from build123d import *

# Parameters (mm, degrees)
SKETCH1_W                      = 81.37
SKETCH1_H                      = 20
SKETCH1_R                      = 2.5
BOSS_EXTRUDE1_DEPTH            = 15
CBORE_FOR_M5_SHCS1_D           = 5.5
CBORE_FOR_M5_SHCS1_CBORE_D     = 10
CBORE_FOR_M5_SHCS1_CBORE_DEPTH = 10
SKETCH8_W                      = 20
SKETCH8_H                      = 15
BOSS_EXTRUDE3_DEPTH            = 8.5
CUT_EXTRUDE1_START             = -3
CUT_EXTRUDE1_DEPTH             = 9
SKETCH7_W                      = 5
SKETCH7_H                      = 6.1
BOSS_EXTRUDE2_DEPTH            = 4
CHAMFER1_SIZE                  = 0.5


with BuildPart() as part:
    # Sketch1 → Boss-Extrude1 (new body)
    with BuildSketch(Plane(origin=(0, 0, 0), x_dir=(1, 0, 0), z_dir=(0, 1, 0))):
        with Locations((-29.315, 0)):
            Rectangle(SKETCH1_W, SKETCH1_H)
        Circle(SKETCH1_R, mode=Mode.SUBTRACT)
        with Locations((-18.03, 0)):
            Circle(SKETCH1_R, mode=Mode.SUBTRACT)
    extrude(amount=BOSS_EXTRUDE1_DEPTH)

    # CBORE for M5 SHCS1 (through all)
    with Locations(Plane(origin=(0, 15, 0), x_dir=(1, 0, 0), z_dir=(0, 1, 0))):
        with Locations((-58, 0), (-38.03, 0)):
            CounterBoreHole(CBORE_FOR_M5_SHCS1_D / 2, CBORE_FOR_M5_SHCS1_CBORE_D / 2, CBORE_FOR_M5_SHCS1_CBORE_DEPTH)

    # Sketch8 → Boss-Extrude3 (add)
    with BuildSketch(Plane(origin=(11.37, 0, 0), x_dir=(0, 0, -1), z_dir=(1, 0, 0))):
        with Locations((0, 7.5)):
            Rectangle(SKETCH8_W, SKETCH8_H)
    extrude(amount=BOSS_EXTRUDE3_DEPTH)

    # Sketch6 → Cut-Extrude1 (cut)
    with BuildSketch(Plane(origin=(0, 15, 0), x_dir=(1, 0, 0), z_dir=(0, 1, 0)).offset(CUT_EXTRUDE1_START)):
        with BuildLine():
            Line((-29.53, 0), (-29.53, -10))
            Line((-29.53, -10), (11.5, -10))
            Line((11.5, -10), (11.5, 0))
            ThreePointArc((11.5, 0), (3.780046296, 10.860996731), (-9.015, 7.140012255))
            ThreePointArc((-9.015, 7.140012255), (-21.810046296, 10.860996731), (-29.53, 0))
        make_face()
    extrude(amount=-CUT_EXTRUDE1_DEPTH, mode=Mode.SUBTRACT)

    # Sketch7 → Boss-Extrude2 (add)
    with BuildSketch(Plane.XZ):
        with Locations((-11.5, 0)):
            Rectangle(SKETCH7_W, SKETCH7_H)
        with Locations((-67.5, 0)):
            Rectangle(SKETCH7_W, SKETCH7_H)
    extrude(amount=BOSS_EXTRUDE2_DEPTH)

    # Chamfer1
    chamfer1_edges = [part.edges().sort_by_distance(p)[0] for p in [
        (-2.5, 15, 0),
        (-70, 15, 0),
        (-20.53, 15, 0),
        (-25.065, 15, 10),
        (-43.03, 15, 0),
        (-63, 15, 0),
        (19.87, 15, 0),
        (-25.065, 15, -10),
    ]]
    chamfer(chamfer1_edges, length=CHAMFER1_SIZE)


solid = part.part
The model under review builds one solid part; all positions refer to its coordinate system, in mm. A direction names the side the tool comes from. Round coordinates to 2 decimals unless told otherwise and drop trailing zeros. Loops run counter-clockwise (first coordinate to the right, second up) from the corner with the lowest first, then second, coordinate; pieces in that order, holes last. Notation, with made-up numbers: M 80,29.25 L 108,29.25 A15 ccw 108,48.25 Z; hole C -15.5,20 d2. An arc over 180 degrees is marked long. Answer as a JSON object with one key per item and string values.
Item 1: Clearance check with flat-ended pins moving along their axes: P1, Ø2, axis at x = -37.5, z = -7.5, coming from the -Y side; P2, Ø4.5, axis at x = -58, z = 0, coming from the +Y side; P3, Ø5, axis at x = -38.5, z = -1.5, coming from the +Y side; P4, Ø3, axis at x = -12.5, y = -2.5, coming from the +Z side. State where each tip first meets the part, or that it passes through.
Check sheet entries:
{"P1": "y = 0", "P2": "through", "P3": "y = 5", "P4": "z = 3.05"}
Item 2: For line 1 along X through (y, z) = (13.55, 0); line 2 along X through (y, z) = (-1.25, -1.5); line 3 along Z through (x, y) = (-18.03, 2.25), list the stretches that pass through material, from the lowest coordinate up.
Check sheet entries:
{"line 1": "-70 to -63, -53 to -43.03, -33.03 to -20.53, -15.53 to -2.5, 2.5 to 19.87", "line 2": "-70 to -65, -14 to -9", "line 3": "-10 to -2.5, 2.5 to 10"}
Item 3: The part is to be moulded in two halves that separate along Y. For faces 1 (the face through (11.5, 8, 5)), 2 (the face through (-10.52, 7.56, -8.71)), 3 (the face through (-14, -2, 0)), 4 (the face through (-12, -4, 0)), say which applies: +Y half, -Y half, draft (parallel to the pull), parting line (faces both ways), or undercut.
Check sheet entries:
{"face 1": "undercut", "face 2": "undercut", "face 3": "draft", "face 4": "-Y half"}
Item 4: We need section C-C, the plane z = 1. State how many separate pieces and enclosed holes the cut face has, and give its area (3 significant figures).
Check sheet entries:
{"separate pieces": "6", "enclosed holes": "0", "area": "715 mm2"}
Item 5: Tool access review of faces 5 (the face through (-68, -2, -3.05)), 6 (the face through (-68, -2, 3.05)), 7 (the face through (-27.9, 7.6, -5.9)), 8 (the face through (-65, -2, 0)), 9 (the face through (-41.715, 9.817, -3.379)): name each direction out of +Z, -Z, +X, -X, +Y, -Y from which nothing blocks a thin tool from reaching the whole face with its end or side.
Check sheet entries:
{"face 5": "-Z, +X, -X, -Y", "face 6": "+Z, +X, -X, -Y", "face 7": "+Z", "face 8": "+Z, -Z, -Y", "face 9": "+Y"}
Item 6: We need section B-B, the plane y = 7. State the section outline as (x, z) points (3 decimals), and give its area (3 significant figures).
Check sheet entries:
{"outline": "M -70,-10 L -23.709,-10 A11.5 cw -29.53,0 L -29.53,10 L -70,10 Z; M -12.351,-10 L -5.679,-10 A11.5 cw -9.015,-7.14 A11.5 cw Z; M 5.679,-10 L 19.87,-10 L 19.87,10 L 11.5,10 L 11.5,0 A11.5 cw Z; hole C -58,0 d10; hole C -38.03,0 d10", "area": "862 mm2"}
Item 7: We need section A-A, the plane x = -58. State the section outline as (y, z) points.
Check sheet entries:
{"outline": "M 0,-10 L 14.5,-10 L 15,-9.5 L 15,-5.5 L 14.5,-5 L 5,-5 L 5,-2.75 L 0,-2.75 Z; M 0,2.75 L 5,2.75 L 5,5 L 14.5,5 L 15,5.5 L 15,9.5 L 14.5,10 L 0,10 Z"}
